Input: part model. Units: mm. Frame: model coordinates. Coordinates: 2 decimals unless noted, no trailing zeros. Write each loop counter-clockwise with the first axis right and the second up, starting at its lowest first coordinate (ties: lowest second). Pieces come first, ordered by that corner, then holes. Notation, with made-up numbers: M 35.5,82.25 L 51.5,82.25 A7 cw 51.5,94.25 Z; hole C 14.25,1.5 d4. An arc over 180 degrees is marked long. Use CSV: the item, a comma, the result in double quotes.
```python
from build123d import *

# Parameters (mm, degrees)
F0_W     = 290
F0_H     = 580
F1_DEPTH = 10
F2_W     = 270
F2_H     = 560
F3_DEPTH = 10
F4_R     = 1


with BuildPart() as f1:
    # F0 (on Top) → F1 (new body)
    with BuildSketch(Plane.XY):
        with Locations((-39.619565, 4.486432)):
            Rectangle(F0_W, F0_H)
    extrude(amount=F1_DEPTH)

    # F2 (on face) → F3 (join)
    with BuildSketch(Plane(origin=(0, 0, 0), x_dir=(1, 0, 0), z_dir=(0, 0, -1))):
        with Locations((-39.619565, -4.486432)):
            Rectangle(F2_W, F2_H)
    extrude(amount=F3_DEPTH)

    # F4
    f4_edges = [f1.edges().sort_by_distance(p)[0] for p in [
        (95.380435, 4.486432, -10),
        (-39.619565, -275.513568, -10),
        (-174.619565, 4.486432, -10),
        (-39.619565, 284.486432, -10),
        (-184.619565, 4.486432, 0),
        (95.380435, -275.513568, -5),
        (-174.619565, -275.513568, -5),
        (-39.619565, -275.513568, 0),
        (95.380435, 284.486432, -5),
        (95.380435, 4.486432, 0),
        (105.380435, -285.513568, 5),
        (105.380435, 294.486432, 5),
        (105.380435, 4.486432, 0),
        (105.380435, 4.486432, 10),
        (-184.619565, -285.513568, 5),
        (-39.619565, -285.513568, 0),
        (-39.619565, -285.513568, 10),
        (-184.619565, 294.486432, 5),
        (-184.619565, 4.486432, 10),
        (-39.619565, 294.486432, 0),
        (-39.619565, 294.486432, 10),
        (-174.619565, 284.486432, -5),
        (-39.619565, 284.486432, 0),
        (-174.619565, 4.486432, 0),
    ]]
    fillet(f4_edges, radius=F4_R)


solid = f1.part
```
1. Contact query for flat-ended pins moving along their axis: pin 1 Ø1 at (x, z) = (-66, -5.5) entering from +Y; pin 2 Ø4 at (y, z) = (-45.5, -6.5) entering from +X; pin 3 Ø4 at (x, z) = (27, -4.5) entering from -Y. Output: stop coordinate, or through.
Resolved:
pin 1,"stops at y = 284.49"
pin 2,"stops at x = 95.38"
pin 3,"stops at y = -275.51"
2. Section A-A (x = -17.5). Return loops of the section in (y, z), then the cut area to 3 significant figures.
Resolved:
outline,"M -285.51,1 A1 ccw -284.51,0 L -276.51,0 A1 cw -275.51,-1 L -275.51,-9 A1 ccw -274.51,-10 L 283.49,-10 A1 ccw 284.49,-9 L 284.49,-1 A1 cw 285.49,0 L 293.49,0 A1 ccw 294.49,1 L 294.49,9 A1 ccw 293.49,10 L -284.51,10 A1 ccw -285.51,9 Z"
area,"11,400 mm^2"
3. Section B-B (y = 29). Return loops of the section in (x, z).
Resolved:
outline,"M -184.62,1 A1 ccw -183.62,0 L -175.62,0 A1 cw -174.62,-1 L -174.62,-9 A1 ccw -173.62,-10 L 94.38,-10 A1 ccw 95.38,-9 L 95.38,-1 A1 cw 96.38,0 L 104.38,0 A1 ccw 105.38,1 L 105.38,9 A1 ccw 104.38,10 L -183.62,10 A1 ccw -184.62,9 Z"
4. Material intervals for line 1 (X direction, y = 149, z = -3.25); line 2 (Y direction, x = -104, z = -5.5); line 3 (Y direction, x = -67.5, z = -0.5), sorted ascending. Write a range as [from, to].
Resolved:
line 1,"x = [-174.62, 95.38]"
line 2,"y = [-275.51, 284.49]"
line 3,"y = [-275.65, 284.62]"
